Input: dimensioned drawing with shaded views. Units: mm. Origin: part minimum x, y, z. A direction names the side the tool comes from. Give positions to 0.01 mm unless a question says otherwise; leave off trailing zeros. Order: outer loops, then holes, each group sorted by start corner. A loop starts at its lowest first (then second) coordinate and runs counter-clockwise, first axis right, second up. Notation, with made-up numbers: (-22, -28.75) - (-2, -28.75) arc R23 ccw to (-2, -9.75) - close; hole circle Ø9 at (59, 11.25). An arc over 180 degrees is marked (long way). Answer as CSV lines item,"result".
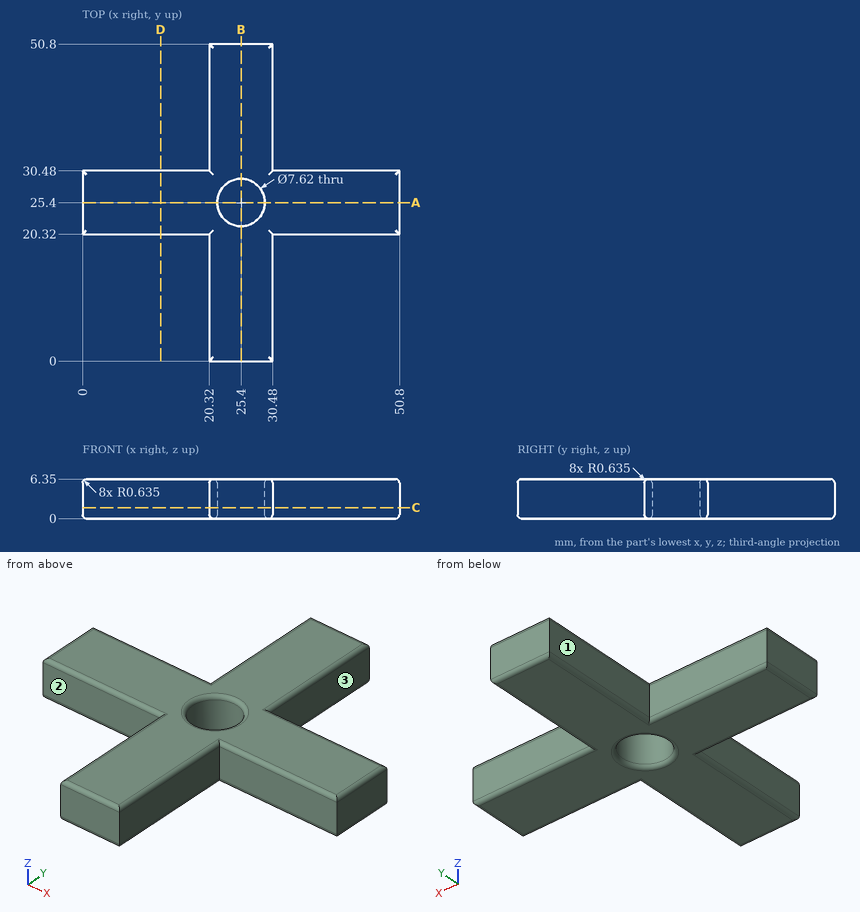
(1) Access query for the marked faces 1, 2 and 3. Directions: +Z, -Z, +X, -X, +Y, -Y. A direction counts if a zero-diameter tool reaches every point of the face in a straight line with its end or side. Return the directions, or none.
Completed:
face 1,"+Z, -Z, -X, +Y"
face 2,"+Z, -Z, -X, -Y"
face 3,"+Z, -Z, +X, +Y"
(2) Cut plane D-D (x = 12.5). Return loops of the section in (y, z) (3 decimals), then the cut area to 3 significant figures.
Completed:
outline,"(20.32, 0.635) arc R0.635 ccw to (20.955, 0) - (29.845, 0) arc R0.635 ccw to (30.48, 0.635) - (30.48, 5.715) arc R0.635 ccw to (29.845, 6.35) - (20.955, 6.35) arc R0.635 ccw to (20.32, 5.715) - close"
area,"64.2 mm²"
(3) Cut plane C-C (z = 1.75). Return loops of the section in (x, y).
Completed:
outline,"(0, 20.32) - (20.32, 20.32) - (20.32, 0) - (30.48, 0) - (30.48, 20.32) - (50.8, 20.32) - (50.8, 30.48) - (30.48, 30.48) - (30.48, 50.8) - (20.32, 50.8) - (20.32, 30.48) - (0, 30.48) - close; hole circle Ø7.62 at (25.4, 25.4)"
(4) Contact query for flat-ended pins moving along their axis: pin 1 (6 mm diameter, centred on x = 25.4, y = 25.4, fed in from +Z); pin 2 (2 mm diameter, centred on x = 17, z = 2, fed in from +Y); pin 3 (1.5 mm diameter, centred on y = 40.5, z = 4, fed in from +X); pin 4 (3 mm diameter, centred on x = 43.5, z = 5, fed in from -Y). Output: stop coordinate, or through.
Completed:
pin 1,"through"
pin 2,"y = 30.48"
pin 3,"x = 30.48"
pin 4,"y = 20.32"
(5) Cut plane A-A (y = 25.4). Return loops of the section in (x, z) (3 decimals).
Completed:
outline,"(0, 0.635) arc R0.635 ccw to (0.635, 0) - (20.955, 0) arc R0.635 ccw to (21.59, 0.635) - (21.59, 5.715) arc R0.635 ccw to (20.955, 6.35) - (0.635, 6.35) arc R0.635 ccw to (0, 5.715) - close; (29.21, 0.635) arc R0.635 ccw to (29.845, 0) - (50.165, 0) arc R0.635 ccw to (50.8, 0.635) - (50.8, 5.715) arc R0.635 ccw to (50.165, 6.35) - (29.845, 6.35) arc R0.635 ccw to (29.21, 5.715) - close"
(6) Ray query, line 1 (X direction, y = 25.4, z = 3.9); line 2 (Y direction, x = 18, z = 4). Return the intervals inside material, ascending. Write a range as from..to.
Completed:
line 1,"0..21.59, 29.21..50.8"
line 2,"20.32..30.48"
